```python
from build123d import *

# Parameters (mm, degrees)
F0_W     = 254
F0_H     = 152.4
F1_DEPTH = 152.4
F2_R     = 101.6
F3_DEPTH = 152.4
F4_W     = 254
F4_H     = 50.8
F5_DEPTH = 76.2


with BuildPart() as f1:
    # F0 (on Top) → F1 (new body)
    with BuildSketch(Plane.XY):
        with Locations((127, 76.2)):
            Rectangle(F0_W, F0_H)
    extrude(amount=F1_DEPTH)

    # F2 (on face) → F3 (cut)
    with BuildSketch(Plane.XZ):
        with Locations((127, 152.4)):
            Circle(F2_R)
    extrude(amount=-F3_DEPTH, mode=Mode.SUBTRACT)

    # F4 (on face) → F5 (cut)
    with BuildSketch(Plane.XZ):
        with Locations((127, 127)):
            Rectangle(F4_W, F4_H)
    extrude(amount=-F5_DEPTH, mode=Mode.SUBTRACT)


solid = f1.part
```
Verification items for the finished model (mm, model axes). A direction names the side the tool comes from. Coordinates: 2 decimals unless noted, no trailing zeros. Order: outer loops, then holes, each group sorted by start corner. A loop starts at its lowest first (then second) coordinate and runs counter-clockwise, first axis right, second up. Notation, with made-up numbers: (-20, 2.25) -> (15, 2.25) arc R20 ccw to (15, 15.25) -> close; hole circle Ø9 at (76.5, -40). An arc over 180 degrees is marked (long way). Put each result on its own line as item: value. Start each with the question number.
1) Go/stop test with flat-tipped pins: pin 1 (1.5 mm diameter, centred on x = 45, y = 111.5, fed in from +Z); pin 2 (2 mm diameter, centred on x = 152, y = 98.5, fed in from +Z); pin 3 (11.5 mm diameter, centred on x = 230, y = 37, fed in from +Z); pin 4 (1 mm diameter, centred on y = 102.5, z = 91, fed in from -X). Record where each tip stops, or that it passes through.
2) Cross-section at D-D (z = 117.5). Enter the section's corners in (x, y).
3) Tool access check on faces 1 (the flat face through (13, 115, 152.4)), 2 (the flat face through (15, 76.2, 127)). Record the directions out of +Z, -Z, +X, -X, +Y, -Y that give a thin tool (end or side, any length) a straight path to the whole face; none if there is none.
4) Material ranges on L1, parallel to Z at x = 19, y = 60; L2, parallel to X at y = 56, z = 95.5; L3, parallel to X at y = 125, z = 137.5, recorded low to high.
5) Release check for a two-part mould opening along X. For faces 3 (the cylindrical face through (124.766, 75.133, 50.825)), 4 (the flat face through (254, 75, 58)), 5 (the flat face through (239, 76.2, 127)), 6 (the flat face through (0, 75, 58)) record: pulls with the +X half, pulls with the -X half, needs draft (parallel to the pull), parting line crosses it, or undercut.
6) Cross-section at C-C (x = 127). Enter the section's corners in (y, z), plus the area to 3 significant figures.
7) Cross-section at B-B (y = 70.5). Enter the section's corners in (x, z), plus the area to 3 significant figures.
8) Cross-section at A-A (z = 80). Enter the section's corners in (x, y), plus the area to 3 significant figures.
Geometry check:
1. pin 1: stops at z = 93.45
1. pin 2: stops at z = 54.18
1. pin 3: stops at z = 101.6
1. pin 4: stops at x = 0
2. outline: (0, 76.2) -> (31.58, 76.2) -> (31.58, 152.4) -> (0, 152.4) -> close; (222.42, 76.2) -> (254, 76.2) -> (254, 152.4) -> (222.42, 152.4) -> close
3. face 1: +Z, +X, -X, +Y, -Y
3. face 2: +Z, +X, -X, -Y
4. L1: z = 0 to 101.6
4. L2: x = 0 to 42.83, 211.17 to 254
4. L3: x = 0 to 26.5, 227.5 to 254
5. face 3: undercut
5. face 4: pulls with the +X half
5. face 5: needs draft
5. face 6: pulls with the -X half
6. outline: (0, 0) -> (152.4, 0) -> (152.4, 50.8) -> (0, 50.8) -> close
6. area: 7,740 mm^2
7. outline: (0, 0) -> (254, 0) -> (254, 101.6) -> (214.99, 101.6) arc R101.6 cw to (39.01, 101.6) -> (0, 101.6) -> close
7. area: 19,500 mm^2
8. outline: (0, 0) -> (55.72, 0) -> (55.72, 152.4) -> (0, 152.4) -> close; (198.28, 0) -> (254, 0) -> (254, 152.4) -> (198.28, 152.4) -> close
8. area: 17,000 mm^2
